Autodesk Inventor part; units mm, degrees
ref_plane "Work Plane1" through (-47.5, 0, 0) normal (1, 0, 0) x (0, 1, 0)
ref_plane "XZ Plane" through (0, 0, 0) normal (0, 1, 0) x (-1, 0, 0)
ref_plane "XY Plane" through (0, 0, 0) normal (0, 0, 1) x (1, 0, 0)
sketch "Sketch1" plane through (0, 0, 0) normal (0, 1, 0) x (-1, 0, 0)
  circle A0 centre (0, 0) radius 47.5
  dimension "d0" = 95
extrude "Extrusion1" add sketch "Sketch1" along normal blind 20
shell "Shell1" thickness 5 removed faces 2 at (-10.3648, 20, 5.7529) at (-10.3648, 0, 5.7529)
sketch "Sketch2" plane through (0, 20, 0) normal (0, 1, 0) x (1, 0, 0)
  line L0 (-62.0625, 51.3519) -> (57.6609, 51.3519)
  line L1 (57.6609, 51.3519) -> (57.6609, 0)
  line L2 (57.6609, 0) -> (-62.0625, 0)
  line L3 (-62.0625, 0) -> (-62.0625, 51.3519)
  point P0 (0, 0)
extrude "Extrusion2" cut sketch "Sketch2" against normal through all
ref_plane "Work Plane1" through (-47.5, 0, 0) normal (1, 0, 0) x (0, 1, 0)
sketch "Sketch3" plane through (-47.5, 0, 0) normal (1, 0, 0) x (0, 1, 0)
  line L0 (0, 0) -> (0, 47.5)
  line L1 (0, 0) -> (20, 0)
  line L2 (20, 0) -> (20, 10)
  line L3 (20, 10) -> (0, 10)
  line L4 (0, 10) -> (0, 0)
  point P0 (0, 10)
  dimension "d7" = 20
  dimension "d8" = 10
extrude "Extrusion3" add sketch "Sketch3" along normal blind 2 and the other way blind 15
mirror "Mirror1" about plane through (0, 0, 0) normal (1, 0, 0) of "Extrusion3"
sketch "Sketch6" plane through (-62.5, 20, 10) normal (0, 0, 1) x (1, 0, 0)
  line L0 (10.3322, -14.0055) -> (5.7134, -13.9945)
  line L1 (5.7134, -13.9945) -> (3.4135, -9.9891)
  line L2 (3.4135, -9.9891) -> (5.7324, -5.9945)
  line L3 (5.7324, -5.9945) -> (10.3512, -6.0055)
  line L4 (10.3512, -6.0055) -> (12.6511, -10.0109)
  line L5 (12.6511, -10.0109) -> (10.3322, -14.0055)
  line L6 (0, -20) -> (0, 0)
  line L7 (16.0646, 0) -> (0, 0)
  point P0 (62.5, -20)
  point P1 (8.0323, -10)
  point P2 (0, -10)
  point P3 (8.0323, 0)
  dimension "d27" = 8
extrude "Extrusion4" cut sketch "Sketch6" against normal blind 5
sketch "Sketch7" plane through (-62.5, 20, 5) normal (0, 0, 1) x (1, 0, 0)
  line L0 (0, -20) -> (0, 0)
  line L1 (16.0646, 0) -> (0, 0)
  point P0 (62.5, -20)
  point P1 (8.0323, -10)
  point P2 (0, -10)
  point P3 (8.0323, 0)
hole "Hole3" at (-54.4677, 10, 5) direction (0, 0, -1) diameter 5.5 end through all
mirror "Mirror3" about plane through (0, 0, 0) normal (1, 0, 0) of "Extrusion4", "Hole3"
fillet "Fillet1" radius 2 23 edges at (-62.5, 0, 5) (-62.5, 20, 5) (-46.4354, 10, 10) (-54.4677, 0, 10) (-62.5, 10, 10) (-54.4677, 20, 10) (0, 20, 47.5) (0, 20, 42.5) (0, 0, 47.5) (-52.5, 20, 0) (52.5, 20, 0) (-62.5, 10, 0) (-52.5, 0, 0) (52.5, 0, 0) (0, 0, 42.5) (54.4677, 20, 10) (62.5, 10, 10) (54.4677, 0, 10) (62.5, 0, 5) (62.5, 20, 5) (62.5, 10, 0) (-42.5, 10, 0) (42.5, 10, 0)
properties part number "ur5e_cable_tube_bottom_85mm"
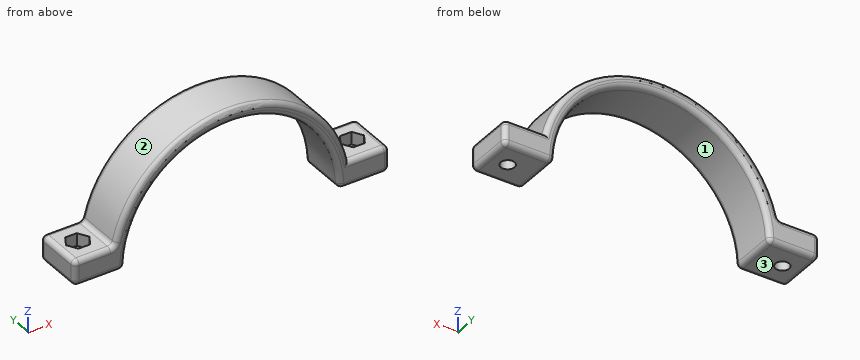
Here's how the part is built. I have some questions about the finished solid (model axes, mm). Face numbers are marked on the shaded views. Give positions to 0.01 mm unless a question says otherwise; leave off trailing zeros. Loops run counter-clockwise (first coordinate to the right, second up) from the corner with the lowest first, then second, coordinate; pieces in that order, holes last. Notation, with made-up numbers: M 24,3.5 L 44,3.5 A29 cw 44,28.5 Z; hole C 71,71 d9. An arc over 180 degrees is marked long. Use one line per item in the form item = value. Start each with the question number.
Q1. If we section it at A-A (x = 0): Write out the boundary of the cut face in (y, z).
Q2. Will these pins go through, and if not, where does the flat tip stop? pin 1 Ø6.5 at (x, y) = (-56.5, 8.5) entering from +Z; pin 2 Ø6 at (x, y) = (-1, 2.5) entering from +Z; pin 3 Ø8 at (x, y) = (4.5, 7.5) entering from -Z; pin 4 Ø5 at (x, y) = (54.47, 10) entering from -Z.
Q3. If we section it at B-B (y = 4.25): Write out the boundary of the cut face in (x, z), then the cut area to 3 significant figures.
Q4. Thinking about a two-plate mould opening in X: for the marked faces 1, 2 and 3, which applies, +X half, -X half, draft (parallel to the pull), parting line (faces both ways), or undercut?
Q5. I need wall thicknesses on line 1 along X through (y, z) = (10, 2.25); line 2 along X through (y, z) = (10, 1.8); line 3 along Z through (x, y) = (-0.5, 5.5). Which ranges of each line are inside material? Lowest first, please.
Taken from the geometry:
q1.outline = M 0,44.5 A2 ccw 2,42.5 L 18,42.5 A2 ccw 20,44.5 L 20,45.5 A2 ccw 18,47.5 L 2,47.5 A2 ccw 0,45.5 Z
q2.pin_1 = 10
q2.pin_2 = 47.5
q2.pin_3 = 41.64
q2.pin_4 = through
q3.outline = M -62.5,2 A2 ccw -60.5,0 L -44.46,0 A2 ccw -42.46,1.91 A42.5 cw 42.46,1.91 A2 ccw 44.46,0 L 60.5,0 A2 ccw 62.5,2 L 62.5,8 A2 ccw 60.5,10 L 46.44,10 A47.5 ccw -46.08,11.52 A2 cw -48.02,10 L -60.5,10 A2 ccw -62.5,8 Z
q3.area = 1,010 mm^2
q4.face_1 = undercut
q4.face_2 = parting line
q4.face_3 = draft
q5.line_1 = -62.5 to -57.22, -51.72 to -42.44, 42.44 to 51.72, 57.22 to 62.5
q5.line_2 = -62.49 to -57.22, -51.72 to -42.47, 42.47 to 51.72, 57.22 to 62.49
q5.line_3 = 42.5 to 47.5
